```python
from build123d import *

# Parameters (mm, degrees)
SKETCH1_R                              = 87.5
BOSS_EXTRUDE1_DEPTH                    = 10
SKETCH2_R                              = 7.5
BOSS_EXTRUDE2_DEPTH                    = 80
CBORE_FOR_M5_HEX_HEAD_BOLT1_AT_2_COUNT = 2
CBORE_FOR_M5_HEX_HEAD_BOLT1_AT_2_PITCH = 113.13708499
CBORE_FOR_M5_HEX_HEAD_BOLT1_AT_3_COUNT = 2
CBORE_FOR_M5_HEX_HEAD_BOLT1_AT_3_PITCH = 160
CBORE_FOR_M5_HEX_HEAD_BOLT1_AT_4_COUNT = 2
CBORE_FOR_M5_HEX_HEAD_BOLT1_AT_4_PITCH = 113.13708499
SKETCH5_R                              = 87.5
CUT_EXTRUDE1_DEPTH                     = 80
FILLET1_R                              = 0.1
CUT_EXTRUDE2_DEPTH                     = 10
CUT_EXTRUDE3_DEPTH                     = 6
CUT_EXTRUDE4_DEPTH                     = 6
CUT_EXTRUDE5_DEPTH                     = 3
SKETCH11_R                             = 1.1
CUT_EXTRUDE6_DEPTH                     = 10
CUT_EXTRUDE7_DEPTH                     = 5
CIRPATTERN1_COUNT                      = 2
CIRPATTERN1_ANGLE                      = 45
CIRPATTERN1_THE_OTHER_WAY_COUNT        = 2
CIRPATTERN1_THE_OTHER_WAY_ANGLE        = 45


with BuildPart() as part:
    # Sketch1 → Boss-Extrude1 (new body)
    with BuildSketch(Plane(origin=(0, 0, 0), x_dir=(1, 0, 0), z_dir=(0, 1, 0))):
        Circle(SKETCH1_R)
    extrude(amount=BOSS_EXTRUDE1_DEPTH)

    # Sketch2 → Boss-Extrude2 (add)
    with BuildSketch(Plane(origin=(0, 10, 0), x_dir=(1, 0, 0), z_dir=(0, 1, 0))):
        with Locations((0, -80)):
            Circle(SKETCH2_R)
        with Locations((-80, 0)):
            Circle(SKETCH2_R)
        with Locations((0, 80)):
            Circle(SKETCH2_R)
        with Locations((80, 0)):
            Circle(SKETCH2_R)
    extrude(amount=BOSS_EXTRUDE2_DEPTH)

    # Sketch4 → CBORE for M5 Hex Head Bolt1 (revolve, cut)
    with BuildSketch(Plane(origin=(80, 0, 0), x_dir=(0, 0, -1), z_dir=(1, 0, 0))):
        Polygon((0, 0), (0, 21.652366702), (2.75, 20), (2.75, 3.58), (6.12, 3.58), (6.12, 0.025), (6.145, 0), align=None)
    cbore_for_m5_hex_head_bolt1 = revolve(axis=Axis((80, -6.35, 0), (0, 1, 0)), mode=Mode.SUBTRACT)

    # CBORE for M5 Hex Head Bolt1 at 2: CBORE for M5 Hex Head Bolt1 ×2
    with Locations(*[Vector(-0.707106781, 0, -0.707106781) * (i * CBORE_FOR_M5_HEX_HEAD_BOLT1_AT_2_PITCH) for i in range(1, CBORE_FOR_M5_HEX_HEAD_BOLT1_AT_2_COUNT)]):
        add(cbore_for_m5_hex_head_bolt1, mode=Mode.SUBTRACT)

    # CBORE for M5 Hex Head Bolt1 at 3: CBORE for M5 Hex Head Bolt1 ×2
    with Locations(*[(-i * CBORE_FOR_M5_HEX_HEAD_BOLT1_AT_3_PITCH, 0, 0) for i in range(1, CBORE_FOR_M5_HEX_HEAD_BOLT1_AT_3_COUNT)]):
        add(cbore_for_m5_hex_head_bolt1, mode=Mode.SUBTRACT)

    # CBORE for M5 Hex Head Bolt1 at 4: CBORE for M5 Hex Head Bolt1 ×2
    with Locations(*[Vector(-0.707106781, 0, 0.707106781) * (i * CBORE_FOR_M5_HEX_HEAD_BOLT1_AT_4_PITCH) for i in range(1, CBORE_FOR_M5_HEX_HEAD_BOLT1_AT_4_COUNT)]):
        add(cbore_for_m5_hex_head_bolt1, mode=Mode.SUBTRACT)

    # Sketch5 → Cut-Extrude1 (cut)
    with BuildSketch(Plane(origin=(0, 10, 0), x_dir=(1, 0, 0), z_dir=(0, 1, 0))):
        Circle(SKETCH5_R)
    extrude(amount=CUT_EXTRUDE1_DEPTH, mode=Mode.SUBTRACT)

    # Fillet1
    fillet1_edges = [part.edges().sort_by_distance(p)[0] for p in [
        (-87.5, 0, 0),
    ]]
    fillet(fillet1_edges, radius=FILLET1_R)

    # Sketch6 → Cut-Extrude2 (cut)
    with BuildSketch(Plane(origin=(0, 10, 0), x_dir=(1, 0, 0), z_dir=(0, 1, 0))):
        with BuildLine():
            Line((10.606601718, 10.606601718), (71.562528419, -50.349324983))
            ThreePointArc((71.562528419, -50.349324983), (61.871843354, -61.871843354), (50.349324983, -71.562528419))
            Line((50.349324983, -71.562528419), (-10.606601718, -10.606601718))
            ThreePointArc((-10.606601718, -10.606601718), (-10.606601718, 10.606601718), (10.606601718, 10.606601718))
        make_face()
    extrude(amount=-CUT_EXTRUDE2_DEPTH, mode=Mode.SUBTRACT)

    # Sketch7 → Cut-Extrude3 (cut)
    with BuildSketch(Plane(origin=(0, 10, 0), x_dir=(1, 0, 0), z_dir=(0, 1, 0))):
        Polygon((-8.485281374, 26.870057685), (-26.870057685, 8.485281374), (-44.547727215, 26.162950904), (-26.162950904, 44.547727215), align=None)
    cut_extrude3 = extrude(amount=-CUT_EXTRUDE3_DEPTH, mode=Mode.SUBTRACT)

    # Sketch8 → Cut-Extrude4 (cut)
    with BuildSketch(Plane.XZ):
        Polygon((-24.721867284, -16.378007266), (-16.378007266, -24.721867284), (-24.721867284, -33.065727302), (-33.065727302, -24.721867284), align=None)
    cut_extrude4 = extrude(amount=-CUT_EXTRUDE4_DEPTH, mode=Mode.SUBTRACT)

    # Sketch10 → Cut-Extrude5 (cut)
    with BuildSketch(Plane(origin=(0, 4, 0), x_dir=(1, 0, 0), z_dir=(0, 1, 0))):
        Polygon((-41.71930009, 28.991378029), (-28.991378029, 41.71930009), (-21.920310217, 34.648232278), (-34.648232278, 21.920310217), align=None)
    cut_extrude5 = extrude(amount=-CUT_EXTRUDE5_DEPTH, mode=Mode.SUBTRACT)

    # Sketch11 → Cut-Extrude6 (cut)
    with BuildSketch(Plane(origin=(0, 4, 0), x_dir=(1, 0, 0), z_dir=(0, 1, 0))):
        with Locations((-26.065370168, 40.914612573)):
            Circle(SKETCH11_R)
        with Locations((-40.914612573, 26.065370168)):
            Circle(SKETCH11_R)
        with Locations((-32.075777808, 17.226535403)):
            Circle(SKETCH11_R)
        with Locations((-17.226535403, 32.075777808)):
            Circle(SKETCH11_R)
    cut_extrude6 = extrude(amount=-CUT_EXTRUDE6_DEPTH, mode=Mode.SUBTRACT)

    # Sketch12 → Cut-Extrude7 (cut)
    with BuildSketch(Plane(origin=(0, 10, 0), x_dir=(1, 0, 0), z_dir=(0, 1, 0))):
        Polygon((-26.870057685, 8.485281374), (-8.485281374, 26.870057685), (-2.828427125, 21.213203436), (-21.213203436, 2.828427125), align=None)
    cut_extrude7 = extrude(amount=-CUT_EXTRUDE7_DEPTH, mode=Mode.SUBTRACT)

    # CirPattern1: Cut-Extrude3, Cut-Extrude4, Cut-Extrude5, Cut-Extrude6, Cut-Extrude7 ×2 about axis
    cirpattern1_axis = Axis((0, 0, 0), (0, 1, 0))
    for i in range(1, CIRPATTERN1_COUNT):
        add(cut_extrude3.rotate(cirpattern1_axis, i * CIRPATTERN1_ANGLE / (CIRPATTERN1_COUNT - 1)), mode=Mode.SUBTRACT)
        add(cut_extrude4.rotate(cirpattern1_axis, i * CIRPATTERN1_ANGLE / (CIRPATTERN1_COUNT - 1)), mode=Mode.SUBTRACT)
        add(cut_extrude5.rotate(cirpattern1_axis, i * CIRPATTERN1_ANGLE / (CIRPATTERN1_COUNT - 1)), mode=Mode.SUBTRACT)
        add(cut_extrude6.rotate(cirpattern1_axis, i * CIRPATTERN1_ANGLE / (CIRPATTERN1_COUNT - 1)), mode=Mode.SUBTRACT)
        add(cut_extrude7.rotate(cirpattern1_axis, i * CIRPATTERN1_ANGLE / (CIRPATTERN1_COUNT - 1)), mode=Mode.SUBTRACT)

    # CirPattern1 the other way: Cut-Extrude3, Cut-Extrude4, Cut-Extrude5, Cut-Extrude6, Cut-Extrude7 ×2 about axis
    cirpattern1_the_other_way_axis = Axis((0, 0, 0), (0, -1, 0))
    for i in range(1, CIRPATTERN1_THE_OTHER_WAY_COUNT):
        add(cut_extrude3.rotate(cirpattern1_the_other_way_axis, i * CIRPATTERN1_THE_OTHER_WAY_ANGLE / (CIRPATTERN1_THE_OTHER_WAY_COUNT - 1)), mode=Mode.SUBTRACT)
        add(cut_extrude4.rotate(cirpattern1_the_other_way_axis, i * CIRPATTERN1_THE_OTHER_WAY_ANGLE / (CIRPATTERN1_THE_OTHER_WAY_COUNT - 1)), mode=Mode.SUBTRACT)
        add(cut_extrude5.rotate(cirpattern1_the_other_way_axis, i * CIRPATTERN1_THE_OTHER_WAY_ANGLE / (CIRPATTERN1_THE_OTHER_WAY_COUNT - 1)), mode=Mode.SUBTRACT)
        add(cut_extrude6.rotate(cirpattern1_the_other_way_axis, i * CIRPATTERN1_THE_OTHER_WAY_ANGLE / (CIRPATTERN1_THE_OTHER_WAY_COUNT - 1)), mode=Mode.SUBTRACT)
        add(cut_extrude7.rotate(cirpattern1_the_other_way_axis, i * CIRPATTERN1_THE_OTHER_WAY_ANGLE / (CIRPATTERN1_THE_OTHER_WAY_COUNT - 1)), mode=Mode.SUBTRACT)


solid = part.part
```
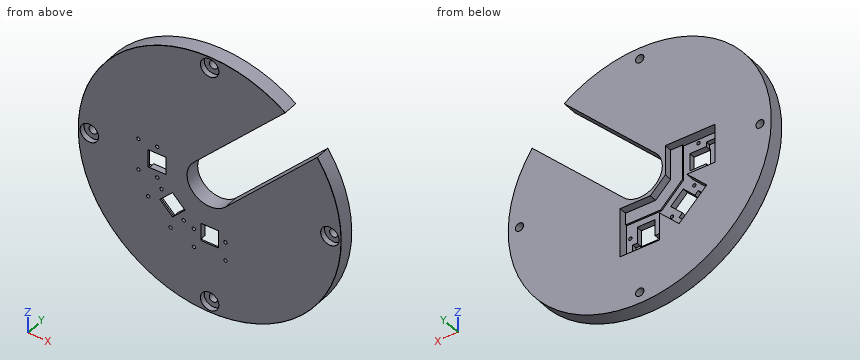
Can you work these out from the model? Positions are in its coordinate system, mm. Round coordinates to 2 decimals unless told otherwise and drop trailing zeros. Loops run counter-clockwise (first coordinate to the right, second up) from the corner with the lowest first, then second, coordinate; pieces in that order, holes last. Notation, with made-up numbers: M 66,68.25 L 121,68.25 A22 ccw 121,92.25 Z; hole C 4,33 d6. An arc over 180 degrees is marked long. Write item = value, one per line. Start each with the question number.
(1) Suppose I cut it at A-A on y = 8. Write out the boundary of the cut face in (x, z).
(2) I need wall thicknesses on line 1 along X through (y, z) = (5.25, -32); line 2 along Z through (x, y) = (10.5, 2.9); line 3 along X through (y, z) = (4.25, 0). Which ranges of each line are inside material? Lowest first, please.
(3) I'm going to push flat-ended pins straight in: P1, Ø1.3, axis at x = -47.362, z = -10.5, coming from the -Y side; P2, Ø1.5, axis at x = -50.5, y = 5.5, coming from the -Z side; P3, Ø2, axis at y = 1.5, z = 0, coming from the -X side; P4, Ø2, axis at y = 4, z = 31, coming from the -X side. Where does each tip first touch, or does it pass through?
(4) Suppose I cut it at B-B on z = 0. Give the number of separate pieces and of enclosed holes in the cut face, plus the area to 3 significant figures.
Answer block:
q1.outline = M -10.61,10.61 L 50.35,71.56 A87.5 ccw long 71.56,50.35 L 10.61,-10.61 A15 cw Z; hole C -80,0 d5.5; hole M -50,-13 L -31.38,-13 L -44.55,-26.16 L -26.16,-44.55 L -13,-31.38 L -13,-50 L 13,-50 L 13,-17 L -7.04,-17 L -17,-7.04 L -17,13 L -50,13 Z; hole C 0,-80 d5.5; hole C 0,80 d5.5; hole C 80,0 d5.5
q2.line_1 = -81.44 to -38.71, -13.62 to -13, 13 to 81.44
q2.line_2 = -86.87 to -48.46, -46.26 to -35.96, -33.76 to -10.71, 31.71 to 86.87
q2.line_3 = -87.5 to -82.75, -77.25 to -50, -25 to -15, 21.21 to 77.25, 82.75 to 87.5
q3.P1 = through
q3.P2 = -71.98
q3.P3 = -87.5
q3.P4 = -82.2
q4.separate_pieces = 5
q4.enclosed_holes = 0
q4.area = 965 mm²
